```python
from build123d import *

# Parameters (mm, degrees)
ESQUISSE1_W               = 105.5
ESQUISSE1_H               = 75
BOSS_EXTRU_1_DEPTH        = 19
ESQUISSE2_R               = 2
ENL_V_MAT_EXTRU_1_DEPTH   = 68.452297959
SYM_TRIE2_COPY_1_SKETCH_R = 2
SYM_TRIE2_COPY_1_DEPTH    = 68.452297959


with BuildPart() as part:
    # Esquisse1 → Boss.-Extru.1 (new body)
    with BuildSketch(Plane.XY):
        Rectangle(ESQUISSE1_W, ESQUISSE1_H)
    extrude(amount=BOSS_EXTRU_1_DEPTH)

    # Esquisse2 → Enlèv. mat.-Extru.1 (cut, through all)
    with BuildSketch(Plane.XY.offset(19)):
        with Locations((-48.25, 33)):
            Circle(ESQUISSE2_R)
    enl_v_mat_extru_1 = extrude(amount=-ENL_V_MAT_EXTRU_1_DEPTH, mode=Mode.SUBTRACT)

    # Symétrie1: Enlèv. mat.-Extru.1 across plane
    add(enl_v_mat_extru_1.mirror(Plane.ZX), mode=Mode.SUBTRACT)

    # Symétrie2: Enlèv. mat.-Extru.1 across plane
    add(enl_v_mat_extru_1.mirror(Plane(origin=(0, 0, 0), x_dir=(0, 0, 1), z_dir=(1, 0, 0))), mode=Mode.SUBTRACT)

    # Symétrie2 copy 1 sketch → Symétrie2 copy 1 (cut, through all)
    with BuildSketch(Plane(origin=(0, 0, 19), x_dir=(-1, 0, 0), z_dir=(0, 0, 1))):
        with Locations((-48.25, 33)):
            Circle(SYM_TRIE2_COPY_1_SKETCH_R)
    extrude(amount=-SYM_TRIE2_COPY_1_DEPTH, mode=Mode.SUBTRACT)


solid = part.part
```
CAD build for the part. Positions are in the model's coordinates, mm. Coordinates: 2 decimals unless noted, no trailing zeros. Write each loop counter-clockwise with the first axis right and the second up, starting at its lowest first coordinate (ties: lowest second). Pieces come first, ordered by that corner, then holes.
(1) Two-plate mould, pull along Y, no slides. Class faces 1 (the face through (-1, -37.5, 9)), 2 (the face through (-52.75, -1, 9)), 3 (the face through (-48.684, 31.048, 9.633)): +Y half, -Y half, draft (parallel to the pull), parting line (faces both ways), or undercut.
(2) Cut at B-B, the plane x = -48.25. List the corners of the cut face in (y, z), and give its area (3 significant figures).
(3) Cut at A-A, the plane y = -33. List the corners of the cut face in (x, z), and give its area (3 significant figures).
(4) Drill centre lines: probe 1 along Y at (x, z) = (-48.25, 11.5); probe 2 along X at (y, z) = (-33, 9.5); probe 3 along X at (y, z) = (34.5, 18.25). Where is each one in solid material? Low to high.
Geometry says:
1. face 1: -Y half
1. face 2: draft
1. face 3: undercut
2. outline: (-37.5, 0) - (-35, 0) - (-35, 19) - (-37.5, 19) - close; (-31, 0) - (31, 0) - (31, 19) - (-31, 19) - close; (35, 0) - (37.5, 0) - (37.5, 19) - (35, 19) - close
2. area: 1,270 mm2
3. outline: (-52.75, 0) - (-50.25, 0) - (-50.25, 19) - (-52.75, 19) - close; (-46.25, 0) - (46.25, 0) - (46.25, 19) - (-46.25, 19) - close; (50.25, 0) - (52.75, 0) - (52.75, 19) - (50.25, 19) - close
3. area: 1,850 mm2
4. probe 1: y = -37.5 to -35, -31 to 31, 35 to 37.5
4. probe 2: x = -52.75 to -50.25, -46.25 to 46.25, 50.25 to 52.75
4. probe 3: x = -52.75 to -49.57, -46.93 to 46.93, 49.57 to 52.75
